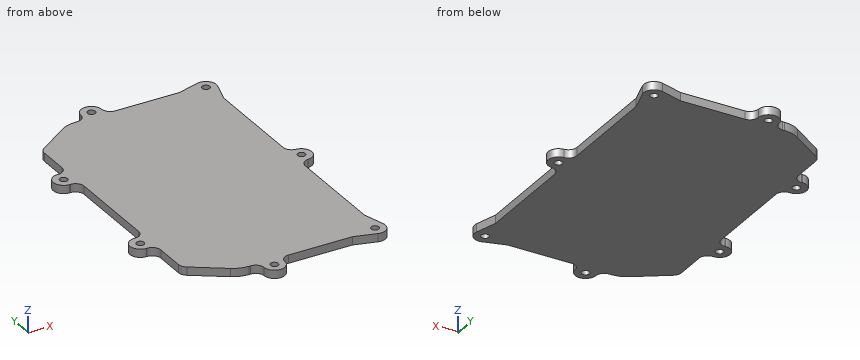
```python
from build123d import *

# Parameters (mm, degrees)
BOSS_EXTRUDE1_DEPTH  = 4.7625
M4_CLEARANCE_HOLE1_D = 4.5


with BuildPart() as part:
    # Sketch1 → Boss-Extrude1 (new body)
    with BuildSketch(Plane.XY):
        with BuildLine():
            Line((-97.832602581, 37.475432296), (-97.832602581, 20.113840969))
            ThreePointArc((-97.832602581, 20.113840969), (-97.214499379, 17.621477955), (-95.503441204, 15.706744322))
            Line((-95.503441204, 15.706744322), (-77.448765904, 3.396738436))
            ThreePointArc((-77.448765904, 3.396738436), (-73.061911597, 1.284058495), (-68.247222211, 0.558335853))
            Line((-68.247222211, 0.558335853), (-67.24507567, 0.558335853))
            ThreePointArc((-67.24507567, 0.558335853), (-63.744637386, -0.87137959), (-62.24605137, -4.342891419))
            ThreePointArc((-62.24605137, -4.342891419), (-56.247222211, -10.224364147), (-50.248393051, -4.342891419))
            ThreePointArc((-50.248393051, -4.342891419), (-48.749807036, -0.87137959), (-45.249368751, 0.558335853))
            Line((-45.249368751, 0.558335853), (-7.916602581, 0.558335853))
            Line((-7.916602581, 0.558335853), (4.631523913, -3.09333052))
            ThreePointArc((4.631523913, -3.09333052), (10.550693091, -1.574959819), (12.069063792, 4.344209359))
            Line((12.069063792, 4.344209359), (8.417397419, 16.892335853))
            Line((8.417397419, 16.892335853), (8.417397419, 75.581748009))
            ThreePointArc((8.417397419, 75.581748009), (9.768409389, 79.000064314), (13.091351964, 80.57110612))
            ThreePointArc((13.091351964, 80.57110612), (18.700097419, 86.558335853), (13.091351964, 92.545565587))
            ThreePointArc((13.091351964, 92.545565587), (9.768409389, 94.116607393), (8.417397419, 97.534923698))
            Line((8.417397419, 97.534923698), (8.417397419, 156.224335853))
            Line((8.417397419, 156.224335853), (12.069063792, 168.772462348))
            ThreePointArc((12.069063792, 168.772462348), (10.550693091, 174.691631526), (4.631523913, 176.210002227))
            Line((4.631523913, 176.210002227), (-7.916602581, 172.558335853))
            Line((-7.916602581, 172.558335853), (-45.249368751, 172.558335853))
            ThreePointArc((-45.249368751, 172.558335853), (-48.749807036, 173.988051296), (-50.248393051, 177.459563126))
            ThreePointArc((-50.248393051, 177.459563126), (-56.247222211, 183.341035853), (-62.24605137, 177.459563126))
            ThreePointArc((-62.24605137, 177.459563126), (-63.744637386, 173.988051296), (-67.24507567, 172.558335853))
            Line((-67.24507567, 172.558335853), (-68.247222211, 172.558335853))
            ThreePointArc((-68.247222211, 172.558335853), (-73.061911597, 171.832613212), (-77.448765904, 169.719933271))
            Line((-77.448765904, 169.719933271), (-95.503441204, 157.409927385))
            ThreePointArc((-95.503441204, 157.409927385), (-97.214499379, 155.495193752), (-97.832602581, 153.002830738))
            Line((-97.832602581, 153.002830738), (-97.832602581, 135.641239411))
            ThreePointArc((-97.832602581, 135.641239411), (-99.297068676, 132.105705505), (-102.832602581, 130.641239411))
            Line((-102.832602581, 130.641239411), (-103.332602581, 130.641239411))
            ThreePointArc((-103.332602581, 130.641239411), (-109.332602581, 124.641239411), (-103.332602581, 118.641239411))
            Line((-103.332602581, 118.641239411), (-102.832602581, 118.641239411))
            ThreePointArc((-102.832602581, 118.641239411), (-99.297068676, 117.176773317), (-97.832602581, 113.641239411))
            Line((-97.832602581, 113.641239411), (-97.832602581, 59.475432296))
            ThreePointArc((-97.832602581, 59.475432296), (-99.297068676, 55.93989839), (-102.832602581, 54.475432296))
            Line((-102.832602581, 54.475432296), (-103.332602581, 54.475432296))
            ThreePointArc((-103.332602581, 54.475432296), (-109.332602581, 48.475432296), (-103.332602581, 42.475432296))
            Line((-103.332602581, 42.475432296), (-102.832602581, 42.475432296))
            ThreePointArc((-102.832602581, 42.475432296), (-99.297068676, 41.010966202), (-97.832602581, 37.475432296))
        make_face()
    extrude(amount=-BOSS_EXTRUDE1_DEPTH)

    # M4 Clearance Hole1 (through all)
    with Locations(Plane(origin=(0, 0, -4.7625), x_dir=(-1, 0, 0), z_dir=(0, 0, -1))):
        with Locations((103.332602581, 48.475432296), (56.247222211, -4.224364147), (-12.700097419, 86.558335853), (56.247222211, 177.341035853), (103.332602581, 124.641239411), (-6.308052404, 2.667680868), (-6.308052404, 170.448990839)):
            Hole(M4_CLEARANCE_HOLE1_D / 2)


solid = part.part
```
For this review, take the finished solid that the model builds, in its own axes (mm). Round coordinates to 2 decimals unless told otherwise and drop trailing zeros. Order: outer loops, then holes, each group sorted by start corner. A loop starts at its lowest first (then second) coordinate and runs counter-clockwise, first axis right, second up. Notation, with made-up numbers: (20.25, 8) -> (55.25, 8) arc R26 cw to (55.25, 45) -> close; hole circle Ø8 at (22.5, 64.25). An arc over 180 degrees is marked (long way). Use a Markdown table: item, result.
Item 1: For line 1 along Y through (x, z) = (7, -0.5); line 2 along Y through (x, z) = (-45.5, -2.8); line 3 along X through (y, z) = (36, -1.05), list the stretches that pass through material, from the lowest coordinate up. Write a range as [from, to].
Resolved:
| item | result |
|---|---|
| line 1 | y = [-3.29, 0.53], [4.81, 168.31], [172.59, 176.41] |
| line 2 | y = [0.55, 172.56] |
| line 3 | x = [-97.83, 8.42] |
Item 2: Take a section at A-A (y = 139.5). State the section outline as (x, z) points, plus the area to 3 significant figures.
Resolved:
| item | result |
|---|---|
| outline | (-97.83, -4.76) -> (8.42, -4.76) -> (8.42, 0) -> (-97.83, 0) -> close |
| area | 506 mm² |
Item 3: For pin 1 (1 mm diameter, centred on x = -42, z = -3, fed in from -Y); pin 2 (1.4 mm diameter, centred on y = 76, z = -3.5, fed in from -X); pin 3 (1.4 mm diameter, centred on y = 115.5, z = -2.5, fed in from +X), all flat-tipped, find the tip position at first contact; note any pin that passes through.
Resolved:
| item | result |
|---|---|
| pin 1 | stops at y = 0.56 |
| pin 2 | stops at x = -97.83 |
| pin 3 | stops at x = 8.42 |
Item 4: Take a section at B-B (x = -3). State the section outline as (y, z) points, plus the area to 3 significant figures.
Resolved:
| item | result |
|---|---|
| outline | (-0.87, -4.76) -> (173.99, -4.76) -> (173.99, 0) -> (-0.87, 0) -> close |
| area | 833 mm² |
Item 5: Take a section at C-C (z = -3.25). State how many separate pieces and enclosed holes the cut face has, plus the area to 3 significant figures.
Resolved:
| item | result |
|---|---|
| separate pieces | 1 |
| enclosed holes | 7 |
| area | 18,500 mm² |
